Verification items for the finished model (mm, model axes). Round coordinates to 2 decimals unless told otherwise and drop trailing zeros. Order: outer loops, then holes, each group sorted by start corner. A loop starts at its lowest first (then second) coordinate and runs counter-clockwise, first axis right, second up. Notation, with made-up numbers: (24, 70.25) -> (63, 70.25) arc R30 cw to (63, 93.25) -> close; hole circle Ø5 at (12, 48). An arc over 180 degrees is marked (long way). Put each result on its own line as item: value.
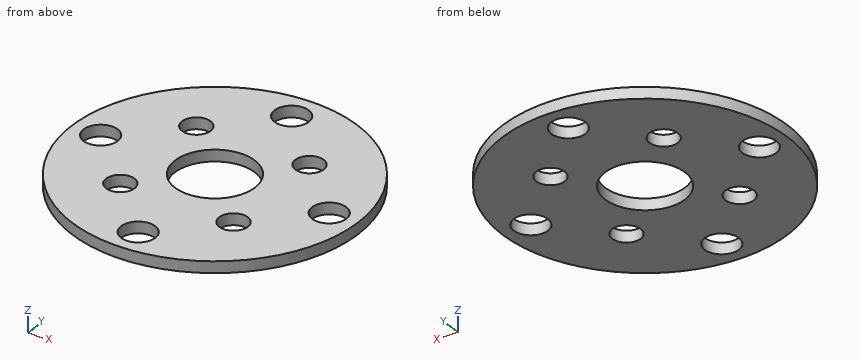
Autodesk Inventor part; units mm, degrees
ref_plane "YZ Plane" through (0, 0, 0) normal (1, 0, 0) x (0, 1, 0)
ref_plane "XZ Plane" through (0, 0, 0) normal (0, 1, 0) x (-1, 0, 0)
ref_plane "XY Plane" through (0, 0, 0) normal (0, 0, 1) x (1, 0, 0)
sketch "Boceto1" plane through (0, 0, 0) normal (0, 0, 1) x (1, 0, 0)
  circle A0 centre (-9.9038, -9.9038) radius 2.5
  circle A1 centre (-9.9038, 9.9038) radius 2.5
  circle A2 centre (-20, 0) radius 3
  circle A3 centre (0, 20) radius 3
  circle A4 centre (20, 0) radius 3
  circle A5 centre (0, -20) radius 3
  circle A6 centre (0, 0) radius 25
  circle A7 centre (0, 0) radius 7
  circle A8 centre (9.9038, 9.9038) radius 2.5
  circle A9 centre (9.9038, -9.9038) radius 2.5
extrude "Extrusión1" add sketch "Boceto1" along normal blind 2
properties part number "_3DPrint"
Item 1: Section check C-C on y = 20. Record the boundary of the cut face in (x, z).
Check sheet entries:
outline: (-15, 0) -> (-3, 0) -> (-3, 2) -> (-15, 2) -> close; (3, 0) -> (15, 0) -> (15, 2) -> (3, 2) -> close
Item 2: Gauge pin test, flat ends, axial feed: pin 1 Ø4.5 at (x, y) = (9.9, 9.9) entering from +Z; pin 2 Ø6 at (x, y) = (6.5, -11) entering from -Z. Record the tip position at first contact, or that the pin passes through.
Check sheet entries:
pin 1: passes through
pin 2: stops at z = 0
Item 3: Material ranges on L1, parallel to Y at x = 0, z = 0.2; L2, parallel to Y at x = 1, z = 0.6; L3, parallel to Y at x = -9.5, z = 1.5, recorded low to high. Write a range as [from, to].
Check sheet entries:
L1: y = [-25, -23], [-17, -7], [7, 17], [23, 25]
L2: y = [-24.98, -22.83], [-17.17, -6.93], [6.93, 17.17], [22.83, 24.98]
L3: y = [-23.12, -12.37], [-7.44, 7.44], [12.37, 23.12]
Item 4: Section check A-A on y = 0. Record the boundary of the cut face in (x, z), then the cut area to 3 significant figures.
Check sheet entries:
outline: (-25, 0) -> (-23, 0) -> (-23, 2) -> (-25, 2) -> close; (-17, 0) -> (-7, 0) -> (-7, 2) -> (-17, 2) -> close; (7, 0) -> (17, 0) -> (17, 2) -> (7, 2) -> close; (23, 0) -> (25, 0) -> (25, 2) -> (23, 2) -> close
area: 48.0 mm^2
